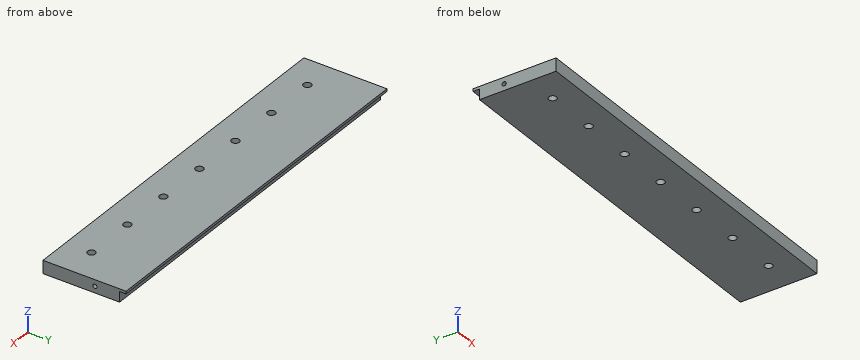
Autodesk Inventor part; units mm, degrees
ref_plane "YZ Plane" through (0, 0, 0) normal (1, 0, 0) x (0, 1, 0)
ref_plane "XZ Plane" through (0, 0, 0) normal (0, 1, 0) x (-1, 0, 0)
ref_plane "XY Plane" through (0, 0, 0) normal (0, 0, 1) x (1, 0, 0)
sketch "Skizze1" plane through (0, 0, 0) normal (0, 0, 1) x (1, 0, 0)
  line L0 (0, 44.8) -> (0, -44.8)
  line L1 (-203, 0) -> (203, 0)
  line L2 (-145, 32) -> (145, 32)
  line L3 (145, 32) -> (145, -32)
  line L4 (145, -32) -> (-145, -32)
  line L5 (-145, -32) -> (-145, 32)
  point P0 (0, 0)
  point P1 (0, 32)
  point P2 (-145, 0)
  dimension "d0" = 290
  dimension "d1" = 64
extrude "Extrusion1" add sketch "Skizze1" along normal blind 10
sketch "Skizze2" plane through (145, -32, 0) normal (1, 0, 0) x (0, 0, -1)
  line L0 (-10, 64) -> (-10, 0)
  line L1 (0, 0) -> (0, 64)
  line L2 (0, 64) -> (-10, 64)
  line L3 (0, 59) -> (-8, 59)
  line L4 (-8, 59) -> (-8, 64)
  point P0 (0, 32)
  dimension "d4" = 2
  dimension "d5" = 5
extrude "Extrusion2" cut sketch "Skizze2" against normal through all
sketch "Skizze3" plane through (0, 0, 10) normal (0, 0, 1) x (1, 0, 0)
  line L0 (-145, -32) -> (-145, 32)
  line L1 (145, -32) -> (-145, -32)
  point P0 (0, 0)
  point P1 (-120, -12)
  dimension "d8" = 25
  dimension "d9" = 20
hole "Bohrung1" at (-120, -12, 10) direction (0, 0, -1) diameter 6 end through all
pattern_linear "Rechteckige Anordnung1" count 7 spacing 40 along (1, 0, 0) of "Bohrung1"
sketch "Skizze4" plane through (145, 27, 8) normal (0, 1, 0) x (1, 0, 0)
  line L0 (-290, 0) -> (-290, 8)
  line L1 (-290, 8) -> (0, 8)
  point P0 (-145, 8)
  point P1 (-265, 4)
  dimension "d20" = 25
  dimension "d21" = 4
hole "Bohrung2" at (-120, 27, 4) direction (0, -1, 0) diameter 2.459 depth 10 tip angle 118
pattern_linear "Rechteckige Anordnung2" count 4 spacing 80 along (1, 0, 0) of "Bohrung2"
sketch "Skizze5" plane through (145, -32, 10) normal (1, 0, 0) x (0, 0, -1)
  line L0 (10, 0) -> (0, 0)
  point P0 (10, 32)
  point P1 (5, 40)
  dimension "d32" = 40
hole "Bohrung3" at (145, 8, 5) direction (-1, 0, 0) diameter 3.242 depth 12 tip angle 118
mirror "Spiegeln1" about plane through (0, 0, 0) normal (1, 0, 0) of "Bohrung3"
properties part number "Tunnelwand" material "Polycarbonate, Clear"
Check sheet for the modelled part. Datum: model origin and axes. Units: mm. Round coordinates to 2 decimals unless told otherwise and drop trailing zeros. Loops run counter-clockwise (first coordinate to the right, second up) from the corner with the lowest first, then second, coordinate; pieces in that order, holes last. Notation, with made-up numbers: M 83,78.5 L 93,78.5 A29 ccw 93,101.5 Z; hole C 64,50 d10. An arc over 180 degrees is marked long. Answer as a JSON object with one key per item and string values.
1. Section check B-B (x = 0). Record the boundary of the cut face in (y, z), plus the area to 3 significant figures.
Reply:
{"outline": "M -32,0 L -15,0 L -15,10 L -32,10 Z; M -9,0 L 27,0 L 27,8 L 32,8 L 32,10 L -9,10 Z", "area": "540 mm²"}
2. Gauge pin test, flat ends, axial feed: P1, Ø1.9, axis at y = 8, z = 5, coming from the +X side; P2, Ø3.5, axis at x = 40, y = -12, coming from the +Z side; P3, Ø1, axis at x = 109, z = 5.5, coming from the +Y side; P4, Ø4, axis at x = -61, y = 30.5, coming from the -Z side. Record the tip position at first contact, or that the pin passes through.
Reply:
{"P1": "stops at x = 132.6", "P2": "passes through", "P3": "stops at y = 27", "P4": "stops at z = 8"}
3. Scan lines: line 1 (Y direction, x = -120, z = 8.5); line 2 (Z direction, x = 140, y = 8); line 3 (X direction, y = 24, z = 4). Record each from-to range of solid material in increasing order.
Reply:
{"line 1": "y = -32 to -15, -9 to 32", "line 2": "z = 0 to 3.38, 6.62 to 10", "line 3": "x = -145 to -121.23, -118.77 to -41.23, -38.77 to 38.77, 41.23 to 118.77, 121.23 to 145"}
4. Section check A-A (y = -12). State how many separate pieces and enclosed holes the cut face has, plus the area to 3 significant figures.
Reply:
{"separate pieces": "8", "enclosed holes": "0", "area": "2,480 mm²"}
5. Section check C-C (x = -93.5). Record the boundary of the cut face in (y, z).
Reply:
{"outline": "M -32,0 L 27,0 L 27,8 L 32,8 L 32,10 L -32,10 Z"}
